Input: part model. Units: mm. Frame: model coordinates. A direction names the side the tool comes from. Round coordinates to 2 decimals unless told otherwise and drop trailing zeros. Write each loop counter-clockwise with the first axis right and the second up, starting at its lowest first coordinate (ties: lowest second). Pieces come first, ordered by that corner, then holes. Notation, with made-up numbers: (-21, -27.75) - (11, -27.75) arc R18 cw to (11, 3.25) - close; hole circle Ø11 at (73.5, -16). An arc over 180 degrees is marked (long way). Use one line per item in the form item = value.
```python
from build123d import *

# Parameters (mm, degrees)
SKETCH1_W           = 250
SKETCH1_H           = 40
SKETCH1_R           = 9.525
BOSS_EXTRUDE1_DEPTH = 38.1
SKETCH3_R           = 15.875
CUT_EXTRUDE1_DEPTH  = 3.175
SKETCH4_R           = 6.35
CUT_EXTRUDE2_DEPTH  = 133.199130103
FILLET1_R           = 2.54


with BuildPart() as part:
    # Sketch1 → Boss-Extrude1 (new body)
    with BuildSketch(Plane(origin=(0, 0, 0), x_dir=(1, 0, 0), z_dir=(0, 1, 0))):
        Rectangle(SKETCH1_W, SKETCH1_H)
        with Locations(Location((-100, 0, 0), (0, 0, 90))):
            Circle(SKETCH1_R, mode=Mode.SUBTRACT)
        with Locations(Location((100, 0, 0), (0, 0, 90))):
            Circle(SKETCH1_R, mode=Mode.SUBTRACT)
    extrude(amount=BOSS_EXTRUDE1_DEPTH)

    # Sketch3 → Cut-Extrude1 (cut)
    with BuildSketch(Plane(origin=(0, 38.1, 0), x_dir=(1, 0, 0), z_dir=(0, 1, 0))):
        with Locations(Location((-100, 0, 0), (0, 0, 270))):
            Circle(SKETCH3_R)
        with Locations(Location((100, 0, 0), (0, 0, 270))):
            Circle(SKETCH3_R)
    extrude(amount=-CUT_EXTRUDE1_DEPTH, mode=Mode.SUBTRACT)

    # Sketch4 → Cut-Extrude2 (cut, through all)
    with BuildSketch(Plane(origin=(0, 38.1, 0), x_dir=(1, 0, 0), z_dir=(0, 1, 0))):
        with Locations(Location((0, 0, 0), (0, 0, 270))):
            Circle(SKETCH4_R)
    extrude(amount=-CUT_EXTRUDE2_DEPTH, mode=Mode.SUBTRACT)

    # Fillet1
    fillet1_edges = [part.edges().sort_by_distance(p)[0] for p in [
        (-100, 34.925, 9.525),
        (100, 34.925, 9.525),
        (0, 38.1, -6.35),
    ]]
    fillet(fillet1_edges, radius=FILLET1_R)


solid = part.part
```
(1) Access query for faces 1 (the face through (-2, 19, -20)), 2 (the face through (-94, 34.925, 11)). Directions: +Z, -Z, +X, -X, +Y, -Y. A direction counts if a zero-diameter tool reaches every point of the face in a straight line with its end or side. Return the directions, or none.
Derived:
face_1 = -Z, +X, -X, +Y, -Y
face_2 = +Y
(2) Cut plane B-B on y = 18.5. Output: boundary loops of the cut face in (x, z) (3 decimals).
Derived:
outline = (-125, -20) - (125, -20) - (125, 20) - (-125, 20) - close; hole circle Ø19.05 at (-100, 0); hole circle Ø12.7 at (0, 0); hole circle Ø19.05 at (100, 0)
(3) Draft query along Z for faces 3 (the face through (106, 34.925, 11)), 4 (the face through (-2, 19, 20)), 5 (the face through (-2, 38.1, -9)), 6 (the face through (-109.444, 15.966, 1.24)). Return one class per face: released by +Z, released by -Z, zero draft, split by the parting line, or undercut.
Derived:
face_3 = undercut
face_4 = released by +Z
face_5 = zero draft
face_6 = undercut
(4) Cut plane A-A on x = 0. Output: boundary loops of the cut face in (y, z).
Derived:
outline = (0, -20) - (38.1, -20) - (38.1, -8.89) arc R2.54 ccw to (35.56, -6.35) - (0, -6.35) - close; (0, 6.35) - (35.56, 6.35) arc R2.54 ccw to (38.1, 8.89) - (38.1, 20) - (0, 20) - close
(5) Material intervals for L1, parallel to X at y = 35, z = 0 (3 decimals); L2, parallel to X at y = 13.5, z = 7; L3, parallel to Z at x = 100, y = 25 (3 decimals), sorted ascending.
Derived:
L1 = -125 to -115.875, -84.125 to -6.35, 6.35 to 84.125, 115.875 to 125
L2 = -125 to -106.46, -93.54 to 93.54, 106.46 to 125
L3 = -20 to -9.525, 9.525 to 20
(6) Cut plane C-C on x = -100. Output: boundary loops of the cut face in (y, z) (3 decimals), then the cut area to 3 significant figures.
Derived:
outline = (0, -20) - (38.1, -20) - (38.1, -15.875) - (34.925, -15.875) - (34.925, -12.065) arc R2.54 ccw to (32.385, -9.525) - (0, -9.525) - close; (0, 9.525) - (32.385, 9.525) arc R2.54 ccw to (34.925, 12.065) - (34.925, 15.875) - (38.1, 15.875) - (38.1, 20) - (0, 20) - close
area = 755 mm^2
(7) Cut plane D-D on z = 2. Count the separate pieces of the cut face and the enclosed holes in it, then the cut area to 3 significant figures.
Derived:
separate_pieces = 4
enclosed_holes = 0
area = 7,560 mm^2
(8) First-contact query: pin 1 Ø14.5 at (x, z) = (0, 0) entering from +Y. Flat tip, straight axial feed; report the tip coordinate or a pass-through.
Derived:
pin_1 = 37.5
